Work out the finished part from the listing and answer in its coordinate system (mm). Face numbers are marked on the shaded views. Give positions to 0.01 mm unless a question says otherwise; leave off trailing zeros. Loops run counter-clockwise (first coordinate to the right, second up) from the corner with the lowest first, then second, coordinate; pieces in that order, holes last.
```python
from build123d import *
from build123d import SkipClean  # not in build123d's __all__

# Parameters (mm, degrees)
F0_R     = 7.5
F1_DEPTH = 40
F2_START = 30
F2_DEPTH = 10
F3_R     = 15
F4_DEPTH = 20
F6_D     = 4.4
F6_DEPTH = 19
F6_TIP   = 1.3218933619


# Not quite as in the source:
# - after a boolean that leaves OpenCascade's solid faulty, fix() repairs it


with BuildPart() as f1:
    # F0 (on Top) → F1 (new body)
    with BuildSketch(Plane.XY):
        with BuildLine():
            ThreePointArc((14.7, -2.9849623113), (14.9248115566, -1.5), (15, 0))
            ThreePointArc((15, 0), (14.9248115566, 1.5), (14.7, 2.9849623113))
            ThreePointArc((14.7, 2.9849623113), (0, 15), (-14.7, 2.9849623113))
            ThreePointArc((-14.7, 2.9849623113), (-15, 0), (-14.7, -2.9849623113))
            ThreePointArc((-14.7, -2.9849623113), (0, -15), (14.7, -2.9849623113))
        make_face()
        Circle(F0_R, mode=Mode.SUBTRACT)
    extrude(amount=F1_DEPTH)

    # F0 (on Top) → F2 (join)
    with BuildSketch(Plane.XY.offset(F2_START)):
        with BuildLine():
            ThreePointArc((-14.7, -2.9849623113), (-15, 0), (-14.7, 2.9849623113))
            ThreePointArc((-14.7, 2.9849623113), (-18, 0), (-14.7, -2.9849623113))
        make_face()
        with BuildLine():
            ThreePointArc((14.7, 2.9849623113), (14.9248115566, 1.5), (15, 0))
            ThreePointArc((15, 0), (14.9248115566, -1.5), (14.7, -2.9849623113))
            ThreePointArc((14.7, -2.9849623113), (18, 0), (14.7, 2.9849623113))
        make_face()
    extrude(amount=F2_DEPTH)

    # F3 (on face) → F4 (join)
    with BuildSketch(Plane(origin=(0, 0, 0), x_dir=(1, 0, 0), z_dir=(0, 0, -1))):
        Circle(F3_R)
    with SkipClean():  # cleaning this boolean's faces spoils the solid; the shape is the same uncleaned
        extrude(amount=F4_DEPTH)

    # F6
    with Locations(Plane(origin=(0, 0, -20), x_dir=(1, 0, 0), z_dir=(0, 0, -1))):
        with Locations((0, 0)):
            Hole(F6_D / 2, depth=F6_DEPTH)
            with Locations((0, 0, -(F6_DEPTH + F6_TIP / 2))):  # 118° drill point
                Cone(0, F6_D / 2, F6_TIP, mode=Mode.SUBTRACT)

    add(f1.part.fix(), mode=Mode.REPLACE)


solid = f1.part
```
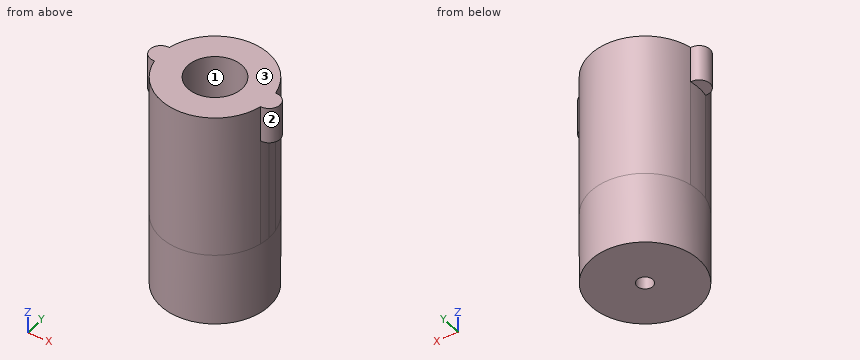
Q1. Consider line 1 along Y through (x, z) = (0, -7.25); line 2 along Z through (x, y) = (-3, 5); line 3 along Z through (x, y) = (-16, 1.5). Determine where each line is inside the solid, lowest interval first.
Q2. Section D-D on y = -5.75 is taken. Give the vertices of the cut face in (x, z).
Q3. Determine the mould class of the marked faces 1, 2 and 3 for opening direction Y: +Y half, -Y half, draft (parallel to the pull), parting line (faces both ways), or undercut.
Q4. Section A-A on z = 23.5 is taken. Give the vertices of the cut face in (x, y).
Q5. Section B-B on x = -4 is taken. Give the vertices of the cut face in (y, z), plus the area to 3 significant figures.
Q6. Given pin 1 (3 mm diameter, centred on y = -4.5, z = 10.5, fed in from +X); pin 2 (1 mm diameter, centred on x = -12, z = 26, fed in from +Y); pin 3 (7.5 mm diameter, centred on x = -1, y = 3, fed in from +Z); pin 4 (3.5 mm diameter, centred on x = 16, y = -1, fed in from -Z), each flat-ended and moving along its own axis, determine where each tip first touches the part or whether it passes through.
Check result:
1. line 1: y = -15 to -2.2, 2.2 to 15
1. line 2: z = -20 to 0
1. line 3: z = 30 to 40
2. outline: (-13.85, -20) - (13.85, -20) - (13.85, 40) - (4.82, 40) - (4.82, 0) - (-4.82, 0) - (-4.82, 40) - (-13.85, 40) - close
3. face 1: undercut
3. face 2: parting line
3. face 3: draft
4. outline: circle Ø30 at (0, 0); hole circle Ø15 at (0, 0)
5. outline: (-14.46, -20) - (14.46, -20) - (14.46, 40) - (6.34, 40) - (6.34, 0) - (-6.34, 0) - (-6.34, 40) - (-14.46, 40) - close
5. area: 1,230 mm2
6. pin 1: stops at x = 14.7
6. pin 2: stops at y = 9.63
6. pin 3: stops at z = 0
6. pin 4: stops at z = -20
